from build123d import *

# Parameters (mm, degrees)
F0_W     = 145
F0_H     = 15
F1_DEPTH = 60
F2_DEPTH = 12
F0_R     = 26
F3_DEPTH = 20
F0_R_2   = 16
F4_DEPTH = 25
F6_DEPTH = 25
F7_DEPTH = 4


with BuildPart() as f1:
    # F0 (on Front) → F1 (new body)
    with BuildSketch(Plane.XZ):
        with Locations((0, -20.210178)):
            Rectangle(F0_W, F0_H)
    extrude(amount=F1_DEPTH)

    # F0 (on Front) → F2 (join)
    with BuildSketch(Plane.XZ):
        with BuildLine():
            Line((12.569365, 87.599361), (-72.5, -12.710178))
            Line((-72.5, -12.710178), (72.5, -12.710178))
            Line((72.5, -12.710178), (72.5, 65.608405))
            ThreePointArc((72.5, 65.608405), (26.787648, 33.689432), (12.569365, 87.599361))
        make_face()
    extrude(amount=F2_DEPTH)

    # F0 (on Front) → F3 (join)
    with BuildSketch(Plane.XZ):
        with BuildLine():
            ThreePointArc((72.5, 65.608405), (50.212352, 97.527377), (12.569365, 87.599361))
            ThreePointArc((12.569365, 87.599361), (26.787648, 33.689432), (72.5, 65.608405))
        make_face()
        with Locations((38.5, 65.608405)):
            Circle(F0_R, mode=Mode.SUBTRACT)
    extrude(amount=F3_DEPTH)

    # F0 (on Front) → F4 (join)
    with BuildSketch(Plane.XZ):
        with Locations((38.5, 65.608405)):
            Circle(F0_R)
        with Locations((38.5, 65.608405)):
            Circle(F0_R_2, mode=Mode.SUBTRACT)
    extrude(amount=F4_DEPTH)

    # F5 (on face) → F6 (cut)
    with BuildSketch(Plane.XY.offset(-12.710178)):
        with BuildLine():
            Line((37.5, -29), (-37.5, -29))
            ThreePointArc((-37.5, -29), (-44.5, -36), (-37.5, -43))
            Line((-37.5, -43), (37.5, -43))
            ThreePointArc((37.5, -43), (44.5, -36), (37.5, -29))
        make_face()
    extrude(amount=-F6_DEPTH, mode=Mode.SUBTRACT)

    # F0 (on Front) → F7 (join)
    with BuildSketch(Plane.XZ):
        with BuildLine():
            ThreePointArc((72.5, 65.608405), (50.212352, 97.527377), (12.569365, 87.599361))
            ThreePointArc((12.569365, 87.599361), (26.787648, 33.689432), (72.5, 65.608405))
        make_face()
        with Locations((38.5, 65.608405)):
            Circle(F0_R, mode=Mode.SUBTRACT)
        with Locations((38.5, 65.608405)):
            Circle(F0_R)
        with Locations((38.5, 65.608405)):
            Circle(F0_R_2, mode=Mode.SUBTRACT)
    extrude(amount=-F7_DEPTH)


solid = f1.part
Check sheet for the modelled part. Datum: model origin and axes. Units: mm. A direction names the side the tool comes from. Give positions to 0.01 mm unless a question says otherwise; leave off trailing zeros. Loops run counter-clockwise (first coordinate to the right, second up) from the corner with the lowest first, then second, coordinate; pieces in that order, holes last. Notation, with made-up numbers: M 81,78.25 L 100,78.25 A16 ccw 100,99.25 Z; hole C 27.25,32.5 d10. An arc over 180 degrees is marked long. Answer as a JSON object with one key per item and string values. Group by question number.
Q1. Access from +Z, -Z, +X, -X, +Y, -Y to the whole of each face (thin tool, end or side, straight path). Record for faces 5 (the flat face through (27, -25, 54)), 6 (the cylindrical face through (52.48, -22.46, 87.53)), 7 (the cylindrical face through (44.5, -36.15, -20.11)), 8 (the flat face through (-1, -25, -12.71)), 9 (the flat face through (-72.5, -30, -20)).
Q2. Cross-section at D-D on x = 62.5. Record the cut outline in (y, z).
Q3. Cross-section at C-C on y = -2. Record the cut outline in (x, z), then the cut area to 3 significant figures.
Q4. Go/stop test with flat-tipped pins: P1, Ø12, axis at x = 56.5, z = -5, coming from the -Y side; P2, Ø1.5, axis at y = -27.5, z = 45.5, coming from the +X side; P3, Ø6, axis at x = 29.5, z = 8.5, coming from the +Y side; P4, Ø14.5, axis at x = -1.5, y = -47.5, coming from the +Z side. Record where each tip stops, or that it passes through.
Q5. Material ranges on line 1 along Z through (x, y) = (38.5, -14.5); line 2 along Z through (x, y) = (38.5, -6.75); line 3 along Z through (x, y) = (38.5, 1.8), recorded low to high. Write a range as [from, to].
Q6. Release check for a two-part mould opening along Z. For faces 1 (the flat face through (-1, -23, -27.71)), 2 (the flat face through (15, -12, 16)), 3 (the flat face through (1, -29, -20)), 4 (the flat face through (-29.37, -5.916, 38.147)) record: released by +Z, released by -Z, zero draft, split by the parting line, or undercut.
Q7. Cross-section at A-A on y = -36. Record the cut outline in (x, z), then the cut area to 3 significant figures.
Q8. Cross-section at B-B on x = -24.5. Record the cut outline in (y, z).
Evaluation:
{
 "1": {"face 5": "+Z, +X, -X, -Y", "face 6": "-Y", "face 7": "+Z, -Z", "face 8": "+X, -X, -Y", "face 9": "+Z, -Z, -X, +Y, -Y"},
 "2": {"outline": "M -60,-27.71 L 0,-27.71 L 0,41.53 L 4,41.53 L 4,89.69 L -20,89.69 L -20,75.61 L -25,75.61 L -25,55.61 L -20,55.61 L -20,41.53 L -12,41.53 L -12,-12.71 L -60,-12.71 Z"},
 "3": {"outline": "M -72.5,-27.71 L 72.5,-27.71 L 72.5,65.61 A34 ccw 12.57,87.6 L -72.5,-12.71 Z; hole C 38.5,65.61 d32", "area": "12,000 mm2"},
 "4": {"P1": "stops at y = -12", "P2": "passes through", "P3": "stops at y = 0", "P4": "stops at z = -12.71"},
 "5": {"line 1": "z = [-27.71, -12.71], [31.61, 49.61], [81.61, 99.61]", "line 2": "z = [-27.71, 49.61], [81.61, 99.61]", "line 3": "z = [31.61, 49.61], [81.61, 99.61]"},
 "6": {"face 1": "released by -Z", "face 2": "undercut", "face 3": "zero draft", "face 4": "released by +Z"},
 "7": {"outline": "M -72.5,-27.71 L -44.5,-27.71 L -44.5,-12.71 L -72.5,-12.71 Z; M 44.5,-27.71 L 72.5,-27.71 L 72.5,-12.71 L 44.5,-12.71 Z", "area": "840 mm2"},
 "8": {"outline": "M -60,-27.71 L -43,-27.71 L -43,-12.71 L -60,-12.71 Z; M -29,-27.71 L 0,-27.71 L 0,43.89 L -12,43.89 L -12,-12.71 L -29,-12.71 Z"}
}
